```python
from build123d import *

# Parameters (mm, degrees)
SKETCH3_R           = 5
BOSS_EXTRUDE2_DEPTH = 332
CUT_EXTRUDE1_START  = -5.5
SKETCH7_R           = 24.093580554
CUT_EXTRUDE1_DEPTH  = 9.55
CUT_EXTRUDE2_START  = 5.5
SKETCH7_2_R         = 24.093580554
CUT_EXTRUDE2_DEPTH  = 9.55


with BuildPart() as part:
    # Sketch3 → Boss-Extrude2 (new body)
    with BuildSketch(Plane.XY):
        Circle(SKETCH3_R)
    extrude(amount=BOSS_EXTRUDE2_DEPTH)

    # Sketch4 → Revolve10 (revolve)
    with BuildSketch(Plane(origin=(0, 0, 0), x_dir=(1, 0, 0), z_dir=(0, 1, 0))):
        with BuildLine():
            ThreePointArc((14.05, -332), (0, -346.05), (-14.05, -332))
            Line((-14.05, -332), (14.05, -332))
        make_face()
    revolve(axis=Axis((-14.05, 0, 332), (1, 0, 0)))

    # Sketch4_6 → Revolve11 (revolve)
    with BuildSketch(Plane(origin=(0, 0, 0), x_dir=(1, 0, 0), z_dir=(0, 1, 0))):
        with BuildLine():
            Line((-14.05, 0), (14.05, 0))
            ThreePointArc((14.05, 0), (0, 14.05), (-14.05, 0))
        make_face()
    revolve(axis=Axis((-14.05, 0, 0), (1, 0, 0)))

    # Sketch8 → Revolve12 (revolve)
    with BuildSketch(Plane(origin=(0, 0, 0), x_dir=(1, 0, 0), z_dir=(0, 1, 0))):
        Polygon((12.29, -6.808700317), (0, -6.808700317), (0, -19.01), (5, -19.01), align=None)
    revolve(axis=Axis((0, 0, 19.01), (0, 0, -1)))

    # Sketch8_3 → Revolve13 (revolve)
    with BuildSketch(Plane(origin=(0, 0, 0), x_dir=(1, 0, 0), z_dir=(0, 1, 0))):
        Polygon((5, -312.99), (0, -312.99), (0, -325.191299683), (12.29, -325.191299683), align=None)
    revolve(axis=Axis((0, 0, 312.99), (0, 0, 1)))

    # Sketch7 → Cut-Extrude1 (cut, through all)
    with BuildSketch(Plane(origin=(0, 0, 0), x_dir=(0, 0, -1), z_dir=(1, 0, 0)).offset(CUT_EXTRUDE1_START)):
        Circle(SKETCH7_R)
        with Locations((-332, 0)):
            Circle(SKETCH7_R)
    extrude(amount=-CUT_EXTRUDE1_DEPTH, mode=Mode.SUBTRACT)

    # Sketch7_2 → Cut-Extrude2 (cut, through all)
    with BuildSketch(Plane(origin=(0, 0, 0), x_dir=(0, 0, -1), z_dir=(1, 0, 0)).offset(CUT_EXTRUDE2_START)):
        Circle(SKETCH7_2_R)
        with Locations((-332, 0)):
            Circle(SKETCH7_2_R)
    extrude(amount=CUT_EXTRUDE2_DEPTH, mode=Mode.SUBTRACT)

    # Sketch6 → Cut-Revolve1 (revolve, cut)
    with BuildSketch(Plane(origin=(0, 0, 0), x_dir=(1, 0, 0), z_dir=(0, 1, 0))):
        with BuildLine():
            Line((-9.5, 0), (9.5, 0))
            ThreePointArc((9.5, 0), (0, 9.5), (-9.5, 0))
        make_face()
    revolve(axis=Axis((-9.5, 0, 0), (1, 0, 0)), mode=Mode.SUBTRACT)

    # Sketch6_3 → Cut-Revolve2 (revolve, cut)
    with BuildSketch(Plane(origin=(0, 0, 0), x_dir=(1, 0, 0), z_dir=(0, 1, 0))):
        with BuildLine():
            Line((-9.5, -332), (9.5, -332))
            ThreePointArc((9.5, -332), (0, -341.5), (-9.5, -332))
        make_face()
    revolve(axis=Axis((-9.5, 0, 332), (1, 0, 0)), mode=Mode.SUBTRACT)


solid = part.part
```
Source: CAD feature listing. Evaluate the final solid. Frame: model axes, mm. A direction names the side the tool comes from. Give positions to 0.01 mm unless a question says otherwise; leave off trailing zeros. Order: outer loops, then holes, each group sorted by start corner. A loop starts at its lowest first (then second) coordinate and runs counter-clockwise, first axis right, second up.
(1) Section query B-B (y = 0). Return the cut outline in (x, z).
(2) Contact query for flat-ended pins moving along their axis: P1, Ø8, axis at y = 4, z = 54, coming from the +X side; P2, Ø1.5, axis at y = 1.5, z = 35.5, coming from the -X side; P3, Ø5, axis at x = -0.5, z = 141.5, coming from the -Y side. Output: stop coordinate, or through.
(3) Section query C-C (z = 276.5). Return the cut outline in (x, y).
(4) Access query for faces 1 (the face through (-5.5, -6, 326)), 2 (the face through (2.8, -5.4, 314.8)). Directions: +Z, -Z, +X, -X, +Y, -Y. A direction counts if a zero-diameter tool reaches every point of the face in a straight line with its end or side. Return the directions, or none.
(5) Section query A-A (x = 0). Return the cut outline in (y, z), plus the area to 3 significant figures.
(6) Pull-direction query (Z, two-part tool) for faces 3 (the face through (-1.08, -4.88, 163.94)), 4 (the face through (5.5, -6, 6)); classes: +Z half, -Z half, draft (parallel to the pull), parting line (faces both ways), or undercut.
(7) Material intervals for line 1 along Z through (x, y) = (-0.75, 2); line 2 along Z through (x, y) = (-4, 1.5); line 3 along Z through (x, y) = (5, -4.5), sorted ascending.
Outcome:
1. outline: (-5.5, -12.93) arc R14.05 ccw to (5.5, -12.93) - (5.5, -7.75) arc R9.5 cw to (-5.5, -7.75) - close; (-5.5, 7.75) arc R9.5 cw to (5.5, 7.75) - (5.5, 18.17) - (5, 19.01) - (5, 312.99) - (5.5, 313.83) - (5.5, 324.25) arc R9.5 cw to (-5.5, 324.25) - (-5.5, 313.83) - (-5, 312.99) - (-5, 19.01) - (-5.5, 18.17) - close; (-5.5, 339.75) arc R9.5 cw to (5.5, 339.75) - (5.5, 344.93) arc R14.05 ccw to (-5.5, 344.93) - close
2. P1: stops at x = 5
2. P2: stops at x = -4.94
2. P3: stops at y = -5
3. outline: circle Ø10 at (0, 0)
4. face 1: +Z, -Z, -X, +Y, -Y
4. face 2: none
5. outline: (-11.82, 7.6) arc R14.05 ccw (long way) to (11.82, 7.6) - (5, 19.01) - (5, 312.99) - (11.82, 324.4) arc R14.05 ccw (long way) to (-11.82, 324.4) - (-5, 312.99) - (-5, 19.01) - close; hole circle Ø19 at (0, 0); hole circle Ø19 at (0, 332)
5. area: 3,780 mm2
6. face 3: undercut
6. face 4: draft
7. line 1: z = -13.89 to -9.26, 9.26 to 322.74, 341.26 to 345.89
7. line 2: z = -13.38 to -8.49, 8.49 to 323.51, 340.49 to 345.38
7. line 3: z = -12.34 to -6.71, 6.71 to 16.12, 315.88 to 325.29, 338.71 to 344.34
